```python
from build123d import *

# Parameters (mm, degrees)
SKETCH1_R           = 1.1303
SKETCH1_W           = 3.2766
SKETCH1_H           = 18.2372
BOSS_EXTRUDE1_DEPTH = 1.5875
FILLET1_R           = 4.445
SKETCH2_W           = 81.9912
SKETCH2_H           = 2.0955
BOSS_EXTRUDE2_DEPTH = 3.175
BOSS_EXTRUDE3_DEPTH = 3.175
SKETCH5_W           = 77.1144
SKETCH5_H           = 0.762
BOSS_EXTRUDE4_DEPTH = 3.175


with BuildPart() as part:
    # Sketch1 → Boss-Extrude1 (new, symmetric)
    with BuildSketch(Plane(origin=(0, 0, 0), x_dir=(1, 0, 0), z_dir=(0, 1, 0))):
        Polygon((-38.5572, -41.9227), (-38.5572, 25.0825), (38.5572, 25.0825), (38.5572, -41.9227), (54.229, -41.9227), (54.229, 41.9227), (-54.229, 41.9227), (-54.229, -41.9227), align=None)
        with Locations(Location((-40.9956, -38.6969, 0), (0, 0, 270))):
            Circle(SKETCH1_R, mode=Mode.SUBTRACT)
        with Locations(Location((-40.9956, 22.3139, 0), (0, 0, 270))):
            Circle(SKETCH1_R, mode=Mode.SUBTRACT)
        with Locations(Location((40.9956, 22.3139, 0), (0, 0, 270))):
            Circle(SKETCH1_R, mode=Mode.SUBTRACT)
        with Locations(Location((40.9956, -38.6969, 0), (0, 0, 270))):
            Circle(SKETCH1_R, mode=Mode.SUBTRACT)
        with Locations((-50.5587, 10.0711)):
            Rectangle(SKETCH1_W, SKETCH1_H, mode=Mode.SUBTRACT)
        with Locations((-50.5587, -17.8689)):
            Rectangle(SKETCH1_W, SKETCH1_H, mode=Mode.SUBTRACT)
        with Locations((50.5587, -17.8689)):
            Rectangle(SKETCH1_W, SKETCH1_H, mode=Mode.SUBTRACT)
        with Locations((50.5587, 10.0711)):
            Rectangle(SKETCH1_W, SKETCH1_H, mode=Mode.SUBTRACT)
        Polygon((-20.5232, 36.6141), (-41.7322, 36.6141), (-41.7322, 39.8907), (-9.5758, 39.8907), (-9.5758, 37.2237), (-9.5758, 36.9697), (1.5748, 36.9697), (1.5748, 28.0289), (-20.5232, 28.0289), align=None, mode=Mode.SUBTRACT)
        Polygon((9.5758, 38.590972839), (9.5758, 39.8907), (39.5478, 39.8907), (39.5478, 37.1221), (44.5262, 37.1221), (44.5262, 30.7721), (35.7632, 30.7721), (35.7632, 36.6141), (9.5758, 36.6141), align=None, mode=Mode.SUBTRACT)
    extrude(amount=BOSS_EXTRUDE1_DEPTH, both=True)

    # Fillet1
    fillet1_edges = [part.edges().sort_by_distance(p)[0] for p in [
        (-54.229, 0, -41.9227),
        (54.229, 0, -41.9227),
        (54.229, 0, 41.9227),
        (-54.229, 0, 41.9227),
    ]]
    fillet(fillet1_edges, radius=FILLET1_R)

    # Sketch2 → Boss-Extrude2 (add)
    with BuildSketch(Plane(origin=(0, 1.5875, 0), x_dir=(1, 0, 0), z_dir=(0, 1, 0))):
        with Locations((0, -40.87495)):
            Rectangle(SKETCH2_W, SKETCH2_H)
    extrude(amount=-BOSS_EXTRUDE2_DEPTH)

    # Sketch4 → Boss-Extrude3 (add, through all)
    with BuildSketch(Plane(origin=(0, 1.5875, 0), x_dir=(1, 0, 0), z_dir=(0, 1, 0))):
        Polygon((35.7632, 36.6141), (39.5478, 36.6141), (39.5478, 37.1221), (44.5262, 37.1221), (44.5262, 30.7721), (35.7632, 30.7721), align=None)
    extrude(amount=-BOSS_EXTRUDE3_DEPTH)

    # Sketch5 → Boss-Extrude4 (add)
    with BuildSketch(Plane(origin=(0, 1.5875, 0), x_dir=(1, 0, 0), z_dir=(0, 1, 0))):
        with Locations((0, -39.4462)):
            Rectangle(SKETCH5_W, SKETCH5_H)
    extrude(amount=-BOSS_EXTRUDE4_DEPTH)


solid = part.part
```
The listing builds one solid part. Answer for the finished solid, in the listing's coordinates (mm). Coordinates: 2 decimals unless noted, no trailing zeros. Loops run counter-clockwise (first coordinate to the right, second up) from the corner with the lowest first, then second, coordinate; pieces in that order, holes last. Notation, with made-up numbers: M -8,-17 L 6,-17 A24 ccw 6,19 Z; hole C 8.5,11 d5. An arc over 180 degrees is marked long. Answer as a JSON object with one key per item and string values. Group by question number.
Item 1: Section C-C (z = -34) is taken. Write down the section's boundary in (x, y).
Item 2: Consider L1, parallel to Z at x = 25.5, y = 1.2; L2, parallel to X at y = 1.3, z = -13; L3, parallel to Z at x = -49, y = 0.75. Determine where each line is inside the solid, lowest interval first.
Item 3: Determine the mould class of faces 1 (the face through (52.197, 0, 18)), 2 (the face through (52.96, 0.02, 40.59)), 3 (the face through (38.557, 0, 7)), 4 (the face through (4, -1.588, -31)) for opening direction X: +X half, -X half, draft (parallel to the pull), parting line (faces both ways), or undercut.
Item 4: Section D-D (x = 24.5) is taken. Write down the section's boundary in (y, z).
Item 5: Section B-B (x = 3) is taken. Write down the section's boundary in (y, z).
Item 6: Section A-A (z = 12.5) is taken. Write down the section's boundary in (x, y), and give its area (3 significant figures).
Item 7: Each of these flat-tipped pins is pushed along its axis until it touches: P1, Ø1.8, axis at x = 41, z = 38.7, coming from the +Y side; P2, Ø1, axis at y = -0.5, z = -38.5, coming from the +X side. Where does it stop, or does it pass through?
Solved:
{
 "1": {"outline": "M -54.23,-1.59 L -20.52,-1.59 L -20.52,1.59 L -54.23,1.59 Z; M 1.57,-1.59 L 54.23,-1.59 L 54.23,1.59 L 1.57,1.59 Z"},
 "2": {"L1": "z = -41.92 to -39.89, -36.61 to -25.08, 39.07 to 41.92", "L2": "x = -54.23 to -52.2, -48.92 to -38.56, 38.56 to 48.92, 52.2 to 54.23", "L3": "z = -41.92 to -19.19, -0.95 to 8.75, 26.99 to 41.92"},
 "3": {"face 1": "undercut", "face 2": "+X half", "face 3": "undercut", "face 4": "draft"},
 "4": {"outline": "M -1.59,-41.92 L 1.59,-41.92 L 1.59,-39.89 L -1.59,-39.89 Z; M -1.59,-36.61 L 1.59,-36.61 L 1.59,-25.08 L -1.59,-25.08 Z; M -1.59,39.07 L 1.59,39.07 L 1.59,41.92 L -1.59,41.92 Z"},
 "5": {"outline": "M -1.59,-41.92 L 1.59,-41.92 L 1.59,-25.08 L -1.59,-25.08 Z; M -1.59,39.07 L 1.59,39.07 L 1.59,41.92 L -1.59,41.92 Z"},
 "6": {"outline": "M -54.23,-1.59 L -52.2,-1.59 L -52.2,1.59 L -54.23,1.59 Z; M -48.92,-1.59 L -38.56,-1.59 L -38.56,1.59 L -48.92,1.59 Z; M 38.56,-1.59 L 48.92,-1.59 L 48.92,1.59 L 38.56,1.59 Z; M 52.2,-1.59 L 54.23,-1.59 L 54.23,1.59 L 52.2,1.59 Z", "area": "78.7 mm2"},
 "7": {"P1": "passes through", "P2": "stops at x = 54.2"}
}
